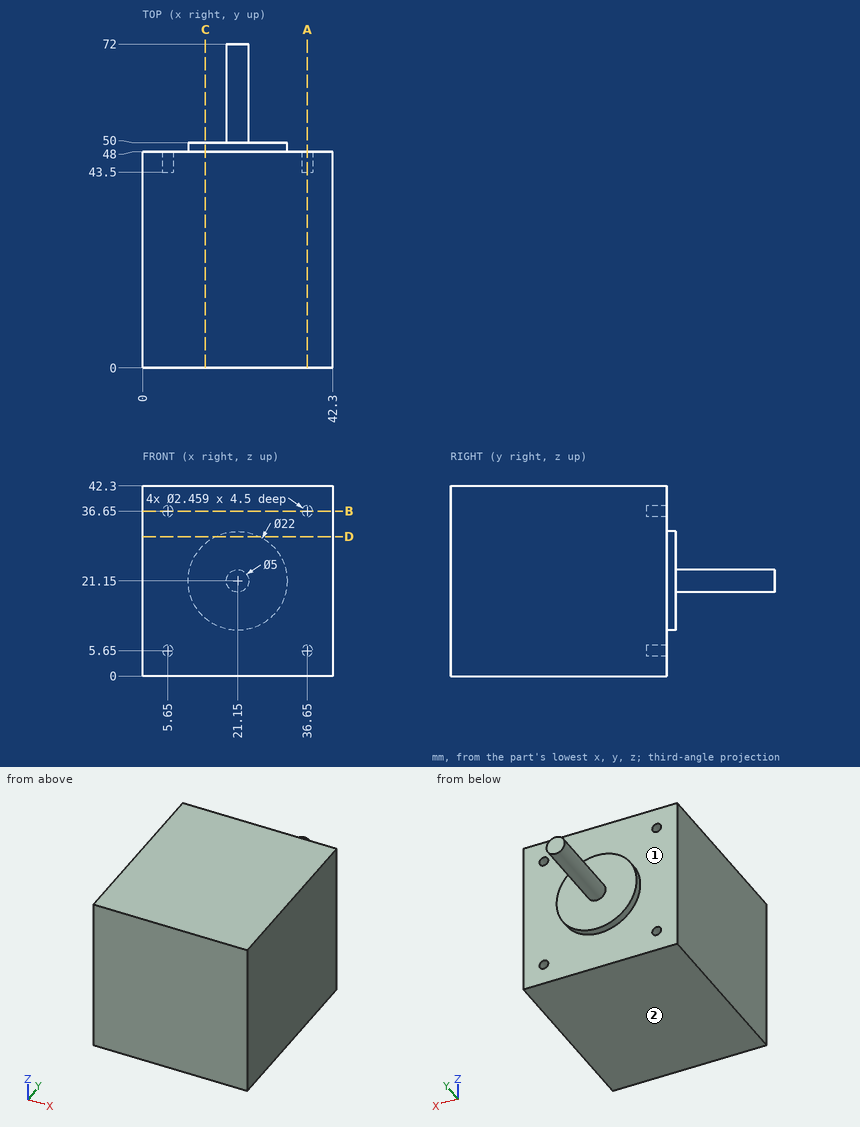
Source: three-view drawing plus pictorial views. Frame: mm from the lowest corner of the part. A direction names the side the tool comes from. Give positions to 0.01 mm unless a question says otherwise; leave off trailing zeros. Loops run counter-clockwise (first coordinate to the right, second up) from the corner with the lowest first, then second, coordinate; pieces in that order, holes last. Notation, with made-up numbers: M 70,-38.5 L 106,-38.5 A21 ccw 106,-27.5 Z; hole C -6,89 d7. An arc over 180 degrees is marked long. Put each result on its own line as item: value.
Q1. Section A-A (x = 36.65). Return the cut outline in (y, z), and give its area (3 significant figures).
Response values:
outline: M 0,0 L 48,0 L 48,4.42 L 43.5,4.42 L 43.5,6.88 L 48,6.88 L 48,35.42 L 43.5,35.42 L 43.5,37.88 L 48,37.88 L 48,42.3 L 0,42.3 Z
area: 2,010 mm²
Q2. Line query: probe 1 along Z at (x, y) = (36.65, 46.65); probe 2 along Z at (x, y) = (36, 46). Output: solid intervals per line, ascending. Write a range as [from, to].
Response values:
probe 1: z = [0, 4.42], [6.88, 35.42], [37.88, 42.3]
probe 2: z = [0, 4.61], [6.69, 35.61], [37.69, 42.3]
Q3. Reachability of the marked faces 1 and 2 from +Z, -Z, +X, -X, +Y, -Y: full face, straight path, thin tool, end or side. Return the list, or none.
Response values:
face 1: +Y
face 2: -Z, +X, -X, +Y, -Y
Q4. Section D-D (z = 31). Return the cut outline in (x, y).
Response values:
outline: M 0,0 L 42.3,0 L 42.3,48 L 26.05,48 L 26.05,50 L 16.25,50 L 16.25,48 L 0,48 Z
Q5. Section B-B (z = 36.65). Return the cut outline in (x, y), and give its area (3 significant figures).
Response values:
outline: M 0,0 L 42.3,0 L 42.3,48 L 37.88,48 L 37.88,43.5 L 35.42,43.5 L 35.42,48 L 6.88,48 L 6.88,43.5 L 4.42,43.5 L 4.42,48 L 0,48 Z
area: 2,010 mm²
Q6. Section C-C (x = 14). Return the cut outline in (y, z).
Response values:
outline: M 0,0 L 48,0 L 48,12.79 L 50,12.79 L 50,29.51 L 48,29.51 L 48,42.3 L 0,42.3 Z
Q7. Pin query (flat end, axial travel): P1, Ø0.7, axis at x = 36, z = 37, coming from the +Y side; P2, Ø1.2, axis at x = 5, z = 5.5, coming from the +Y side. Return the tip coordinate at first contact, or that it passes through.
Response values:
P1: stops at y = 43.5
P2: stops at y = 48
